Autodesk Inventor part; units mm, degrees
ref_plane "YZ Plane" through (0, 0, 0) normal (1, 0, 0) x (0, 1, 0)
ref_plane "XZ Plane" through (0, 0, 0) normal (0, 1, 0) x (-1, 0, 0)
ref_plane "XY Plane" through (0, 0, 0) normal (0, 0, 1) x (1, 0, 0)
sketch "Sketch1" plane through (0, 0, 0) normal (0, 1, 0) x (-1, 0, 0)
  circle A0 centre (-23.8125, 0) radius 2.54
  circle A1 centre (-11.9063, 20.6222) radius 2.54
  circle A2 centre (11.9062, 20.6222) radius 2.54
  circle A3 centre (23.8125, 0) radius 2.54
  circle A4 centre (-11.9063, -20.6222) radius 2.54
  circle A5 centre (11.9062, -20.6222) radius 2.54
  circle A6 centre (0, 0) radius 30.1625
  arc A7 (-1, 3.873) -> (1, 3.873) centre (0, 0) ccw
  line L0 (1, 3.873) -> (1, 5)
  line L1 (1, 5) -> (-1, 5)
  line L2 (-1, 5) -> (-1, 3.873)
  dimension "d0" = 5.08
  dimension "d6" = 5.08
  dimension "d8" = 5.08
  dimension "d10" = 5.08
  dimension "d11" = 60.325
  dimension "d15" = 8
  dimension "d19" = 1
  dimension "d20" = 1
  dimension "d22" = 0
  dimension "d23" = 1
extrude "Extrusion2" add sketch "Sketch1" along normal blind 3.175
properties part number "Pneumatic Hub" material "Aluminum 6061"
Check sheet for the modelled part. Datum: model origin and axes. Units: mm. A direction names the side the tool comes from. Round coordinates to 2 decimals unless told otherwise and drop trailing zeros. Order: outer loops, then holes, each group sorted by start corner. A loop starts at its lowest first (then second) coordinate and runs counter-clockwise, first axis right, second up. Notation, with made-up numbers: (53, -40) -> (68, -40) arc R24 ccw to (68, -27) -> close; hole circle Ø4 at (28, 34). An arc over 180 degrees is marked (long way). One line per item, written item: value. Start each with the question number.
Q1. Cross-section at A-A (x = 0). Record the boundary of the cut face in (y, z) (1 decimal).
Q2. Set-up check for faces 4 (the face through (0, 3.175, -6)), 5 (the face through (0, 2, 5)): record each of +Z, -Z, +X, -X, +Y, -Y from which the full face is reachable in a straight line by a thin tool's end or side.
Q3. Cross-section at D-D (x = 22). Record the boundary of the cut face in (y, z) (3 decimals), and give its area (3 significant figures).
Q4. Cross-section at C-C (y = 1.45). Record the boundary of the cut face in (x, z) (1 decimal).
Q5. Cross-section at B-B (z = 0). Record the boundary of the cut face in (x, y) (1 decimal).
Q6. Gauge pin test, flat ends, axial feed: pin 1 Ø1.6 at (x, y) = (0, 1.5) entering from -Z; pin 2 Ø4 at (x, z) = (-11.91, -20.62) entering from -Y (1 decimal); pin 3 Ø0.9 at (y, z) = (1.5, 4.5) entering from -X; pin 4 Ø1 at (y, z) = (1.5, 16.5) entering from -X. Record the tip position at first contact, or that the pin passes through.
Q7. Mould release check, pull along Z, two halves, no side actions. Record for faces 1 (the face through (12.24, 1.57, -23.14)), 2 (the face through (30.133, 1.565, -1.326)), 3 (the face through (0, 0, -6)): pulls with the +Z half, pulls with the -Z half, needs draft (parallel to the pull), parting line crosses it, or undercut.
Q8. Thickness scan on line 1 (Z direction, x = 0, y = 0.85); line 2 (X direction, y = 3.05, z = -22); line 3 (X direction, y = 1.25, z = -21). Record the ranges inside material, lowest first.
Completed:
1. outline: (0, -30.2) -> (3.2, -30.2) -> (3.2, -4) -> (0, -4) -> close; (0, 5) -> (3.2, 5) -> (3.2, 30.2) -> (0, 30.2) -> close
2. face 4: +Z, -Z, +X, -X, +Y
2. face 5: +Y, -Y
3. outline: (0, -20.634) -> (3.175, -20.634) -> (3.175, -1.779) -> (0, -1.779) -> close; (0, 1.779) -> (3.175, 1.779) -> (3.175, 20.634) -> (0, 20.634) -> close
3. area: 120 mm²
4. outline: circle Ø60.3 at (0, 0); hole circle Ø5.1 at (-23.8, 0); hole circle Ø5.1 at (-11.9, -20.6); hole circle Ø5.1 at (-11.9, 20.6); hole (-1, 3.9) arc R4 ccw (long way) to (1, 3.9) -> (1, 5) -> (-1, 5) -> close; hole circle Ø5.1 at (11.9, -20.6); hole circle Ø5.1 at (11.9, 20.6); hole circle Ø5.1 at (23.8, 0)
5. outline: (-30.2, 0) -> (-26.4, 0) -> (-26.4, 3.2) -> (-30.2, 3.2) -> close; (-21.3, 0) -> (-4, 0) -> (-4, 3.2) -> (-21.3, 3.2) -> close; (4, 0) -> (21.3, 0) -> (21.3, 3.2) -> (4, 3.2) -> close; (26.4, 0) -> (30.2, 0) -> (30.2, 3.2) -> (26.4, 3.2) -> close
6. pin 1: stops at z = -30.16
6. pin 2: passes through
6. pin 3: stops at x = -29.89
6. pin 4: stops at x = -25.57
7. face 1: undercut
7. face 2: parting line crosses it
7. face 3: needs draft
8. line 1: z = -30.16 to -4, 5 to 30.16
8. line 2: x = -20.63 to -14.04, -9.77 to 9.77, 14.04 to 20.63
8. line 3: x = -21.65 to -14.42, -9.39 to 9.39, 14.42 to 21.65
